Could you check a few things on this model? Use its own coordinates, in mm. A direction names the side the tool comes from. Give positions to 0.01 mm unless a question says otherwise; leave off trailing zeros. Write each loop counter-clockwise with the first axis right and the second up, starting at its lowest first coordinate (ties: lowest second). Pieces come first, ordered by that corner, then holes. Notation, with made-up numbers: M 82,6 L 128,6 A31 ccw 128,31 Z; hole C 88.25,-23 d3. An arc over 180 degrees is marked long. Use one line per item in the form item = value.
from build123d import *

# Parameters (mm, degrees)
EXTRUDE_THIN1_DEPTH     = 16
BOSS_EXTRUDE2_DEPTH     = 16
FILLET1_R               = 1
CUT_EXTRUDE2_DEPTH      = 18.058758847
CUT_EXTRUDE2_DEPTH_BACK = 18.058758847


# Read off the part's stored shape, not the designer's step: Imported1
with BuildPart() as part:
    # Sketch2 → Extrude-Thin1 (new, symmetric)
    with BuildSketch(Plane.XY):
        with BuildLine():
            Line((-4.282991407, -1.199997312), (-2.45293323, -1.69036477))
            ThreePointArc((-2.45293323, -1.69036477), (-0.24999913, 2.688e-06), (-2.45293323, 1.690370147))
            Line((-2.45293323, 1.690370147), (-4.282991407, 1.200002688))
            Line((-4.282991407, 1.200002688), (-4.800634272, 3.131853062))
            Line((-4.800634272, 3.131853062), (-2.970575647, 3.62222064))
            ThreePointArc((-2.970575647, 3.62222064), (1.75000087, 2.688e-06), (-2.970575649, -3.622215263))
            Line((-2.970575649, -3.622215263), (-4.800634272, -3.131847685))
            Line((-4.800634272, -3.131847685), (-4.282991407, -1.199997312))
        make_face()
    extrude(amount=EXTRUDE_THIN1_DEPTH, both=True)

    # Sketch4 → Boss-Extrude2 (add, symmetric)
    with BuildSketch(Plane.XY):
        with BuildLine():
            Line((2.602765718, -3.74999537), (2.602765718, 3.659682334))
            Line((2.602765718, 3.659682334), (-1.925829051, 3.749267219))
            ThreePointArc((-1.925829051, 3.749267219), (1.749817484, -0.037083193), (-1.999997188, -3.74999537))
            Line((-1.999997188, -3.74999537), (2.602765718, -3.74999537))
        make_face()
    extrude(amount=BOSS_EXTRUDE2_DEPTH, both=True)

    # Fillet1
    fillet1_edges = [part.edges().sort_by_distance(p)[0] for p in [
        (-4.800634272, 3.131853062, 0),
        (-4.800634272, -3.131847685, 0),
    ]]
    fillet(fillet1_edges, radius=FILLET1_R)

    # Sketch3 → Cut-Extrude2 (cut, two sides: drawn at the far end of the back side and taken through both)
    with BuildSketch(Plane(origin=(0, 0, 0), x_dir=(1, 0, 0), z_dir=(0, 1, 0)).offset(-CUT_EXTRUDE2_DEPTH_BACK)):
        with BuildLine():
            Line((2.738864814, 13.342061251), (2.738864814, 18.762901752))
            Line((2.738864814, 18.762901752), (-4.800634272, 18.762901752))
            Line((-4.800634272, 18.762901752), (-4.800634272, 13.342061251))
            ThreePointArc((-4.800634272, 13.342061251), (-1.030884729, 16), (2.738864814, 13.342061251))
        make_face()
        with BuildLine():
            Line((-4.800634272, -18.762901752), (-4.800634272, -13.342061251))
            ThreePointArc((-4.800634272, -13.342061251), (-1.030884729, -16), (2.738864814, -13.342061251))
            Line((2.738864814, -13.342061251), (2.738864814, -18.762901752))
            Line((2.738864814, -18.762901752), (-4.800634272, -18.762901752))
        make_face()
    extrude(amount=CUT_EXTRUDE2_DEPTH + CUT_EXTRUDE2_DEPTH_BACK, mode=Mode.SUBTRACT)


solid = part.part
1) Thinking about a two-plate mould opening in Y: for faces 1 (the cylindrical face through (-0.25, -0.04, 0.22)), 2 (the flat face through (-3.397, -3.508, 0.217)), 3 (the cylindrical face through (-2.46, 3.72, 0.22)), which applies, released by +Y, released by -Y, zero draft, split by the parting line, or undercut?
Checked values:
face_1 = undercut
face_2 = released by -Y
face_3 = released by +Y
2) I want a section at B-B, the plane y = 2.75. Please give me the cut outline in (x, z).
Checked values:
outline = M -4.52,-13.96 A4 ccw 2.6,-13.68 L 2.6,13.68 A4 ccw -4.52,13.96 Z
3) I want a section at A-A, the plane z = 2. Please give me the cut outline in (x, y), plus the area to 3 significant figures.
Checked values:
outline = M -4.54,-2.17 A1 ccw -3.83,-3.39 L -2.97,-3.62 A3.75 ccw -2,-3.75 L 2.6,-3.75 L 2.6,3.66 L -1.93,3.75 A3.75 ccw -2.97,3.62 L -3.83,3.39 A1 ccw -4.54,2.17 L -4.28,1.2 L -2.45,1.69 A1.75 cw long -2.45,-1.69 L -4.28,-1.2 Z
area = 39.5 mm2
4) For pin 1 Ø1 at (x, y) = (0.5, -2) entering from +Z; pin 2 Ø3 at (x, z) = (1.5, 11.5) entering from +Y, each with a flat end and sliding along its axis, tell me the tip position at first contact or that it passes through.
Checked values:
pin_1 = 15.86
pin_2 = 3.71
5) For faces 4 (the flat face through (-4.414, -1.69, 0.201)), 5 (the flat face through (-3.38, -1.44, 0.22)), 6 (the flat face through (-3.409, 3.505, 0.217)), which set-ups out of +Z, -Z, +X, -X, +Y, -Y let a thin tool reach every point of the face, with its end or its side?
Checked values:
face_4 = +Z, -Z, -X
face_5 = +Z, -Z
face_6 = +Z, -Z, -X, +Y
6) If I drill on L1, parallel to Y at x = 2.25, z = 0; L2, parallel to Y at x = -0.5, z = 12; L3, parallel to Y at x = -1, z = 2, over which ranges is the centre line in solid material (lowest first)?
Checked values:
L1 = -3.75 to 3.67
L2 = -3.75 to -0.9, 0.9 to 3.72
L3 = -3.75 to -1.44, 1.44 to 3.73
7) I want a section at C-C, the plane x = 1.5. Please give me the cut outline in (y, z), plus the area to 3 significant figures.
Checked values:
outline = M -3.75,-15.1 L 3.68,-15.1 L 3.68,15.1 L -3.75,15.1 Z
area = 224 mm2
